The listing builds one solid part. Answer for the finished solid, in the listing's coordinates (mm). Face numbers are marked on the shaded views. A direction names the side the tool comes from. Give positions to 0.01 mm unless a question says otherwise; leave off trailing zeros. Order: outer loops, then holes, each group sorted by start corner. A loop starts at its lowest first (then second) coordinate and runs counter-clockwise, first axis right, second up. Notation, with made-up numbers: (-39.5, 73) - (15.5, 73) arc R24 ccw to (15.5, 102) - close; hole circle Ø7 at (38.25, 68). An arc over 180 degrees is marked (long way). Use CSV: the item, a comma, the result in double quotes.
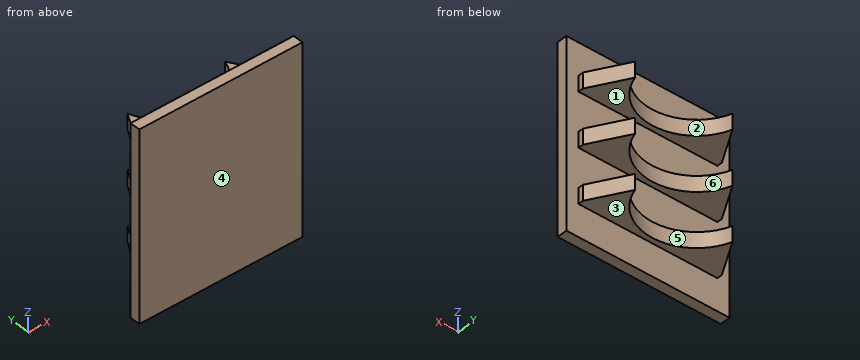
```python
from build123d import *

# Parameters (mm, degrees)
EXTRUDE_1_DEPTH        = 15
PATTERN_LINEAR_1_COUNT = 3
PATTERN_LINEAR_1_PITCH = 52.5
SKETCH_2_W             = 160.09172752
SKETCH_2_H             = 181.978003312
EXTRUDE_2_DEPTH        = 10


with BuildPart() as part:
    # Sketch 1 → Extrude 1 (new body)
    with BuildSketch(Plane.XY):
        with BuildLine():
            Line((-47.784051252, 35.279794638), (-68.152850184, 0))
            Line((-68.152850184, 0), (-68.152850184, -5))
            Line((-68.152850184, -5), (68.152850184, -5))
            Line((68.152850184, -5), (68.152850184, 0))
            Line((68.152850184, 0), (47.784051252, 35.279794638))
            ThreePointArc((47.784051252, 35.279794638), (0, 0), (-47.784051252, 35.279794638))
        make_face()
    extrude(amount=EXTRUDE_1_DEPTH)


with BuildPart() as pattern_linear_1_1:
    # Pattern Linear 1: pattern copy
    add(part.part.moved(Location(Vector(0, 0, 1) * (1 * PATTERN_LINEAR_1_PITCH))))


with BuildPart() as pattern_linear_1_2:
    # Pattern Linear 1: pattern copy
    add(part.part.moved(Location(Vector(0, 0, 1) * (2 * PATTERN_LINEAR_1_PITCH))))


with BuildPart() as part_1:
    add(part.part)

    add(pattern_linear_1_1.part)  # Extrude 2 merges Pattern Linear 1_1

    add(pattern_linear_1_2.part)  # Extrude 2 merges Pattern Linear 1_2
    # Sketch 2 → Extrude 2 (add)
    with BuildSketch(Plane(origin=(0, -5, 0), x_dir=(-1, 0, 0), z_dir=(0, -1, 0))):
        with Locations((0, -60)):
            Rectangle(SKETCH_2_W, SKETCH_2_H)
    extrude(amount=EXTRUDE_2_DEPTH)


solid = part_1.part
```
Item 1: Find the intervals of material crossed by line 1 along Z through (x, y) = (-66, -2.5); line 2 along Y through (x, z) = (-36, 33); line 3 along X through (y, z) = (-1.5, 118), in increasing order.
Taken from the geometry:
line 1,"0 to 15, 52.5 to 67.5, 105 to 120"
line 2,"-15 to -5"
line 3,"-68.15 to 68.15"
Item 2: Which of the six approach directions +Z, -Z, +X, -X, +Y, -Y give full straight-line access (tool end or side, diameter ignored) to the marked faces 1, 2 and 3?
Taken from the geometry:
face 1,"+X, -X, +Y"
face 2,"+Z, -Z, +Y"
face 3,"-Z, +X, -X, +Y"
Item 3: The mould has two halves that part along X. Classify the marked faces 4, 5 and 6: +X half, -X half, draft (parallel to the pull), parting line (faces both ways), or undercut.
Taken from the geometry:
face 4,"draft"
face 5,"undercut"
face 6,"undercut"
Item 4: Each of these flat-tipped pins is pushed along its axis until it touches: pin 1 (4 mm diameter, centred on y = -1.5, z = 115.5, fed in from -X); pin 2 (20 mm diameter, centred on x = -12, y = 9, fed in from -Z); pin 3 (1.5 mm diameter, centred on x = -41, z = 29.5, fed in from +Y). Where does it stop, or does it pass through?
Taken from the geometry:
pin 1,"x = -68.15"
pin 2,"z = 0"
pin 3,"y = -5"
Item 5: The part is cut by section A-A (z = 109). Give the vertices of the cut face in (x, y).
Taken from the geometry:
outline,"(-80.05, -15) - (80.05, -15) - (80.05, -5) - (68.15, -5) - (68.15, 0) - (47.78, 35.28) arc R50 cw to (-47.78, 35.28) - (-68.15, 0) - (-68.15, -5) - (-80.05, -5) - close"
Item 6: The part is cut by section C-C (x = 42.5). Give the vertices of the cut face in (y, z), and give its area (3 significant figures).
Taken from the geometry:
outline,"(-15, -30.99) - (-5, -30.99) - (-5, 0) - (23.66, 0) - (23.66, 15) - (-5, 15) - (-5, 52.5) - (23.66, 52.5) - (23.66, 67.5) - (-5, 67.5) - (-5, 105) - (23.66, 105) - (23.66, 120) - (-5, 120) - (-5, 150.99) - (-15, 150.99) - close"
area,"3,110 mm^2"
Item 7: The part is cut by section D-D (y = 20). Give the vertices of the cut face in (x, z).
Taken from the geometry:
outline,"(-56.61, 0) - (-40, 0) - (-40, 15) - (-56.61, 15) - close; (-56.61, 52.5) - (-40, 52.5) - (-40, 67.5) - (-56.61, 67.5) - close; (-56.61, 105) - (-40, 105) - (-40, 120) - (-56.61, 120) - close; (40, 0) - (56.61, 0) - (56.61, 15) - (40, 15) - close; (40, 52.5) - (56.61, 52.5) - (56.61, 67.5) - (40, 67.5) - close; (40, 105) - (56.61, 105) - (56.61, 120) - (40, 120) - close"
Item 8: The part is cut by section B-B (y = 6.5). Give the vertices of the cut face in (x, z), and give its area (3 significant figures).
Taken from the geometry:
outline,"(-64.4, 0) - (-24.65, 0) - (-24.65, 15) - (-64.4, 15) - close; (-64.4, 52.5) - (-24.65, 52.5) - (-24.65, 67.5) - (-64.4, 67.5) - close; (-64.4, 105) - (-24.65, 105) - (-24.65, 120) - (-64.4, 120) - close; (24.65, 0) - (64.4, 0) - (64.4, 15) - (24.65, 15) - close; (24.65, 52.5) - (64.4, 52.5) - (64.4, 67.5) - (24.65, 67.5) - close; (24.65, 105) - (64.4, 105) - (64.4, 120) - (24.65, 120) - close"
area,"3,580 mm^2"
